Part model, mm, in its own coordinate system. Face numbers are marked on the shaded views. Round coordinates to 2 decimals unless told otherwise and drop trailing zeros. Write each loop counter-clockwise with the first axis right and the second up, starting at its lowest first coordinate (ties: lowest second). Pieces come first, ordered by that corner, then holes. Notation, with made-up numbers: (77, 40) -> (99, 40) arc R6 cw to (99, 51) -> close; hole circle Ø2 at (74, 3.5). An arc over 180 degrees is marked (long way). Return JSON: item names as keys, results as strings. Group by question number.
(1) Saw through at B-B (x = -118). List the corners of the cut face in (y, z), plus the area to 3 significant figures.
(2) Saw through at A-A (z = 12.5). List the corners of the cut face in (x, y), plus the area to 3 significant figures.
(3) Drop flat-ended pins along their axis: pin 1 Ø1 at (x, y) = (-27, -144.5) entering from +Z; pin 2 Ø8 at (y, z) = (-21.5, 157.5) entering from +X; pin 3 Ø3 at (y, z) = (-157, -20.5) entering from -X. Give the stop position or say it passes through.
(4) Saw through at C-C (z = 163.5). List the corners of the cut face in (x, y), plus the area to 3 significant figures.
(5) Drill centre lines: L1, parallel to X at y = 44.5, z = -48.5; L2, parallel to Y at x = -187, z = -57.5; L3, parallel to X at y = 62, z = 51. Where is each one in solid material? Low to high. Write a range as from..to.
(6) Mould opens along X. For the marked faces 1, 2, 3 and 4 say: +X half, -X half, draft (parallel to the pull), parting line (faces both ways), or undercut.
from build123d import *


# Not quite as in the source:
# - the program builds the solid bodies; features that only make, move or delete a surface that nothing else refers to are left out


with BuildPart() as f2:
    # F2: sweep along a path in F1
    with BuildLine(Plane.XY) as f2_path:
        Line((131.5030422138, 92.3344379031), (131.5030422138, -98.4952900969))
        Line((131.5030422138, -98.4952900969), (-316.1564137862, -98.4952900969))
        Line((-316.1564137862, -98.4952900969), (-316.6663944721, 91.8979942799))
    # F0 (on Front) → F2 (sweep)
    with BuildSketch(Plane.XZ):
        with BuildLine():
            Line((223.829728, 92.340303), (197.316539, 92.340303))
            ThreePointArc((197.316539, 92.340303), (223.829728, 118.853492), (197.316539, 145.366681))
            Line((197.316539, 145.366681), (197.316539, 172.683461))
            ThreePointArc((197.316539, 172.683461), (178.0008290346, 180.6842900346), (170, 200))
            Line((170, 200), (170, -200))
            Line((170, -200), (223.829728, -200))
            Line((223.829728, -200), (223.829728, 92.340303))
        make_face()
    sweep(path=f2_path.line, transition=Transition.RIGHT)


solid = f2.part
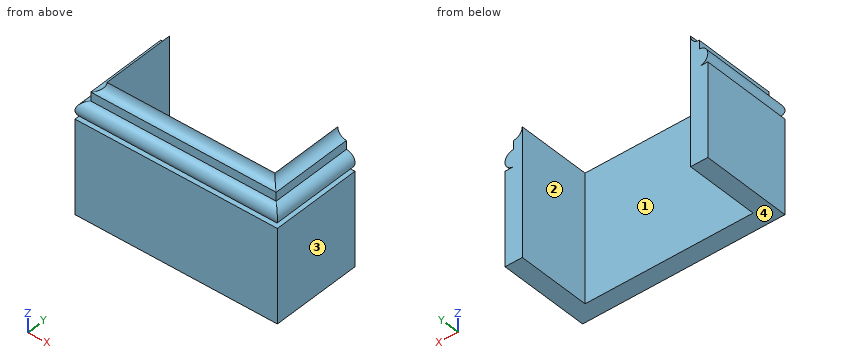
Computed values:
{
 "1": {"outline": "(-190.82, -200) -> (-136.99, -200) -> (-136.99, 200) arc R27.32 cw to (-164.31, 172.68) -> (-164.31, 145.37) arc R26.51 ccw to (-164.31, 92.34) -> (-190.82, 92.34) -> close", "area": "19,200 mm2"},
 "2": {"outline": "(-408.99, 91.65) -> (-408.24, -190.82) -> (223.83, -190.82) -> (223.83, 92.33) -> (170, 92.33) -> (170, -136.99) -> (-354.55, -136.99) -> (-355.16, 91.79) -> close", "area": "58,700 mm2"},
 "3": {"pin 1": "z = 181.73", "pin 2": "x = 197.32", "pin 3": "x = -408.33"},
 "4": {"outline": "(-382.48, 91.72) -> (-381.79, -164.31) -> (197.32, -164.31) -> (197.32, 92.33) -> (170, 92.33) -> (170, -136.99) -> (-354.55, -136.99) -> (-355.16, 91.79) -> close", "area": "28,300 mm2"},
 "5": {"L1": "-408.87..-355.04, 170..223.83", "L2": "-190.82..-136.99", "L3": "-408.91..-355.08, 170..223.83"},
 "6": {"face 1": "undercut", "face 2": "undercut", "face 3": "+X half", "face 4": "draft"}
}
